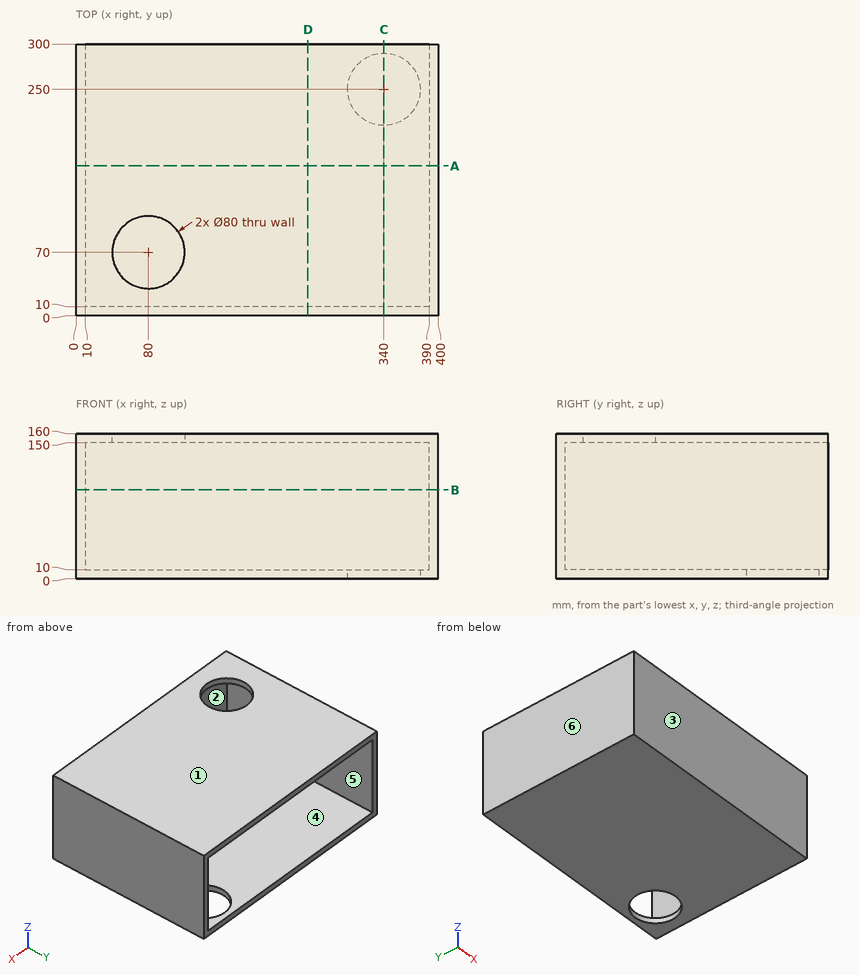
Here's the drawing with two shaded views (mm, measured from the low corner). I have some questions. A direction names the side the tool comes from. Coordinates: 2 decimals unless noted, no trailing zeros. Loops run counter-clockwise (first coordinate to the right, second up) from the corner with the lowest first, then second, coordinate; pieces in that order, holes last. Notation, with made-up numbers: (15.25, 13.25) -> (71.25, 13.25) arc R18 cw to (71.25, 48.25) -> close; hole circle Ø9 at (66.5, 57.25). An arc over 180 degrees is marked (long way). Put each result on its own line as item: value. Start each with the question number.
Q1. I want a section at D-D (x = 256). Write out the boundary of the cut face in (y, z).
Q2. I want a section at B-B (z = 98). Write out the boundary of the cut face in (x, y).
Q3. If I drill on line 1 (X direction, y = 98, z = 14); line 2 (Z direction, x = 258.5, y = 21); line 3 (Y direction, x = 80, z = 157.25), over which ranges is the centre line in solid material (lowest first)? Write a range as [from, to].
Q4. For the marked faces 1 and 2, which set-ups out of +Z, -Z, +X, -X, +Y, -Y let a thin tool reach every point of the face, with its end or its side?
Q5. I'm going to push a flat-ended pin straight in: P1, Ø10, axis at x = 190.5, z = 115.5, coming from the +Y side. Where does the tip first touch, or does it pass through?
Q6. Thinking about a two-plate mould opening in X: for the marked faces 3, 4, 5 and 6, which applies, pulls with the +X half, pulls with the -X half, needs draft (parallel to the pull), parting line crosses it, or undercut?
Q7. I want a section at C-C (x = 340). Write out the boundary of the cut face in (y, z).
Q8. I want a section at A-A (y = 165.5). Write out the boundary of the cut face in (x, z), plus the area to 3 significant figures.
Taken from the geometry:
1. outline: (0, 0) -> (300, 0) -> (300, 10) -> (10, 10) -> (10, 150) -> (300, 150) -> (300, 160) -> (0, 160) -> close
2. outline: (0, 0) -> (400, 0) -> (400, 300) -> (390, 300) -> (390, 10) -> (10, 10) -> (10, 300) -> (0, 300) -> close
3. line 1: x = [0, 10], [390, 400]
3. line 2: z = [0, 10], [150, 160]
3. line 3: y = [0, 30], [110, 300]
4. face 1: +Z, +X, -X, +Y, -Y
4. face 2: +Y
5. P1: stops at y = 10
6. face 3: needs draft
6. face 4: undercut
6. face 5: undercut
6. face 6: pulls with the -X half
7. outline: (0, 0) -> (210, 0) -> (210, 10) -> (10, 10) -> (10, 150) -> (300, 150) -> (300, 160) -> (0, 160) -> close; (290, 0) -> (300, 0) -> (300, 10) -> (290, 10) -> close
8. outline: (0, 0) -> (400, 0) -> (400, 160) -> (0, 160) -> close; hole (10, 10) -> (390, 10) -> (390, 150) -> (10, 150) -> close
8. area: 10,800 mm2
